Geometry check sheet. Reference: drawing and pictorial views, mm from the part's lowest x, y, z. Round coordinates to 2 decimals unless told otherwise and drop trailing zeros. Order: outer loops, then holes, each group sorted by start corner. A loop starts at its lowest first (then second) coordinate and runs counter-clockwise, first axis right, second up. Notation, with made-up numbers: (76, 60) -> (91, 60) arc R21 ccw to (91, 92) -> close; hole circle Ø4 at (82, 54). An arc over 180 degrees is marked (long way). Put each result on its own line as item: value.
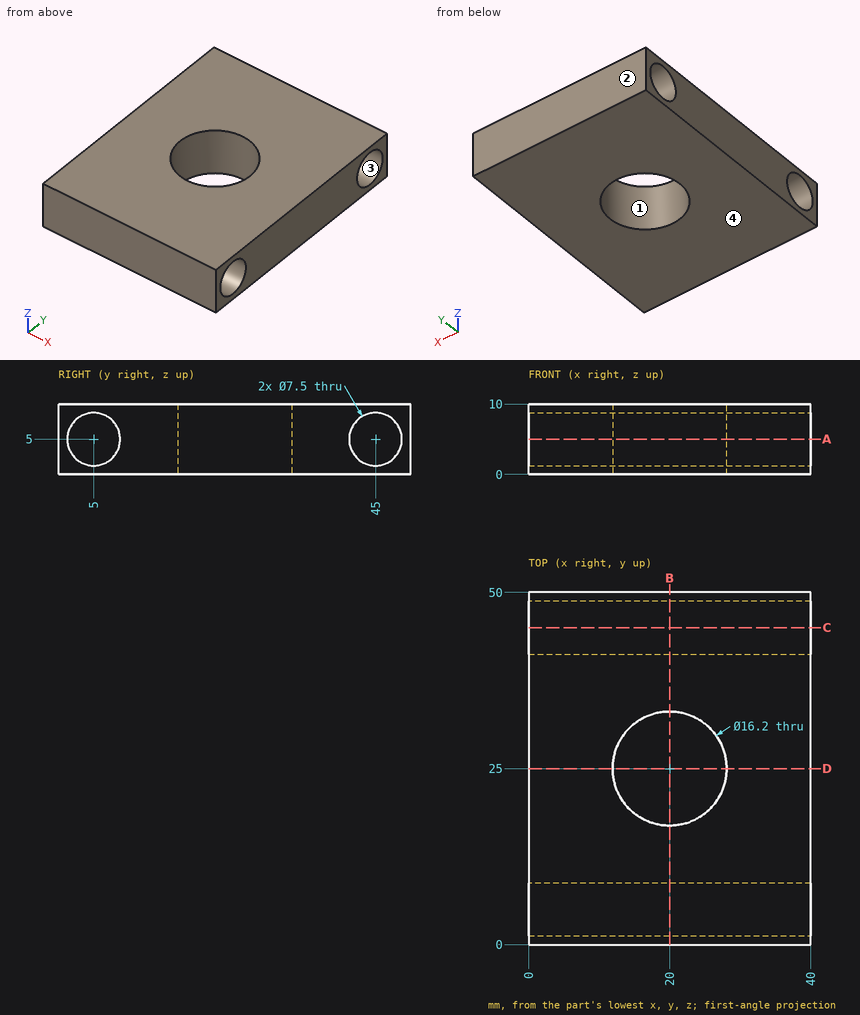
Item 1: Depth check by flat-ended pin: pin 1 Ø1.5 at (x, y) = (25.5, 10.5) entering from -Z. Enter the tip coordinate at first touch or a pass-through.
Geometry check:
pin 1: z = 0
Item 2: Sectioned sample at A-A, the plane z = 5. Record the boundary of the cut face in (x, y), then the cut area to 3 significant figures.
Geometry check:
outline: (0, 0) -> (40, 0) -> (40, 1.25) -> (0, 1.25) -> close; (0, 8.75) -> (40, 8.75) -> (40, 41.25) -> (0, 41.25) -> close; (0, 48.75) -> (40, 48.75) -> (40, 50) -> (0, 50) -> close; hole circle Ø16.2 at (20, 25)
area: 1,190 mm2
Item 3: Sectioned sample at C-C, the plane y = 45. Record the boundary of the cut face in (x, z).
Geometry check:
outline: (0, 0) -> (40, 0) -> (40, 1.25) -> (0, 1.25) -> close; (0, 8.75) -> (40, 8.75) -> (40, 10) -> (0, 10) -> close
Item 4: Sectioned sample at D-D, the plane y = 25. Record the boundary of the cut face in (x, z), then the cut area to 3 significant figures.
Geometry check:
outline: (0, 0) -> (11.9, 0) -> (11.9, 10) -> (0, 10) -> close; (28.1, 0) -> (40, 0) -> (40, 10) -> (28.1, 10) -> close
area: 238 mm2
Item 5: Release check for a two-part mould opening along Y. For the marked faces 1, 2, 3 and 4 record: pulls with the +Y half, pulls with the -Y half, needs draft (parallel to the pull), parting line crosses it, or undercut.
Geometry check:
face 1: undercut
face 2: pulls with the +Y half
face 3: undercut
face 4: needs draft
Item 6: Sectioned sample at B-B, the plane x = 20. Record the boundary of the cut face in (y, z).
Geometry check:
outline: (0, 0) -> (16.9, 0) -> (16.9, 10) -> (0, 10) -> close; (33.1, 0) -> (50, 0) -> (50, 10) -> (33.1, 10) -> close; hole circle Ø7.5 at (5, 5); hole circle Ø7.5 at (45, 5)
Item 7: Material ranges on line 1 along Y through (x, z) = (35, 5.25); line 2 along Y through (x, z) = (20, 5.5); line 3 along Y through (x, z) = (28.5, 2.75), recorded low to high.
Geometry check:
line 1: 0 to 1.26, 8.74 to 41.26, 48.74 to 50
line 2: 0 to 1.28, 8.72 to 16.9, 33.1 to 41.28, 48.72 to 50
line 3: 0 to 2, 8 to 42, 48 to 50
